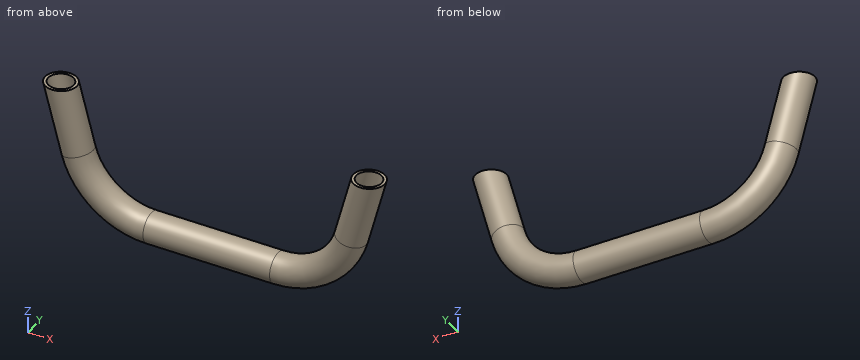
```python
from build123d import *

# Parameters (mm, degrees)
F2_R          = 10
F2_R_2        = 8
F4_W          = 386.4285405924
F4_H          = 84.6193959536
F5_DEPTH      = 10.0010001
F5_DEPTH_BACK = 10.0010001


with BuildPart() as f3:
    # F3: sweep along a path in F0
    with BuildLine(Plane.XZ) as f3_path:
        Line((26.7949192431, 100), (9.9299419155, 37.0590477449))
        ThreePointArc((9.9299419155, 37.0590477449), (-7.9282779485, 10.3323329854), (-38.3663493989, 0))
        Line((-38.3663493989, 0), (-121.7617798121, 0))
        ThreePointArc((-121.7617798121, 0), (-152.1998512625, 10.3323329854), (-170.0580711265, 37.0590477449))
        Line((-170.0580711265, 37.0590477449), (-186.9230484541, 100))
    # F2 (on line) → F3 (sweep)
    with BuildSketch(Plane(origin=(26.7949192431, 0, 100), x_dir=(0.9659258263, 0, -0.2588190451), z_dir=(0.2588190451, 0, 0.9659258263))):
        Circle(F2_R)
        Circle(F2_R_2, mode=Mode.SUBTRACT)
    sweep(path=f3_path.line)

    # F4 (on Front) → F5 (cut, two sides)
    with BuildSketch(Plane.XZ) as f5_sk:
        with Locations((-98.1307812035, 122.3096979768)):
            Rectangle(F4_W, F4_H)
    extrude(amount=-F5_DEPTH, mode=Mode.SUBTRACT)
    extrude(f5_sk.sketch, amount=F5_DEPTH_BACK, mode=Mode.SUBTRACT)


solid = f3.part
```
Part model, mm, in its own coordinate system. Give positions to 0.01 mm unless a question says otherwise; leave off trailing zeros. Order: outer loops, then holes, each group sorted by start corner. A loop starts at its lowest first (then second) coordinate and runs counter-clockwise, first axis right, second up. Notation, with made-up numbers: M 77.5,6.5 L 124.5,6.5 A21 cw 124.5,37.5 Z; hole C 22.5,52.25 d7. An arc over 180 degrees is marked long. Use a Markdown table: item, result. Add a question column.
(1) Saw through at C-C, the plane z = 16.5. Give the number of separate pieces and of enclosed holes in the cut face, and give its area (3 significant figures).
(2) Saw through at A-A, the plane y = 2. Give the cut face in (x, z), and give its area (3 significant figures).
(3) Drop flat-ended pins along their axis: P1, Ø6, axis at y = 5, z = 44, coming from the +X side; P2, Ø9.5, axis at y = 0, z = 0, coming from the -X side; P3, Ø3, axis at y = -6, z = 34, coming from the +X side. Give the stop position or say it passes through.
(4) Probe line 1 along Z through (x, y) = (-67.5, 0); line 2 along Y through (x, z) = (-9.5, 8.5); line 3 along X through (y, z) = (1.25, 32). List the from-to ranges inside material, lowest first. Write a range as [from, to].
(5) Saw through at B-B, the plane x = -70. Give the cut face in (y, z).
Answer key:
| question | item | result |
|---|---|---|
| 1 | separate pieces | 2 |
| 1 | enclosed holes | 2 |
| 1 | area | 318 mm^2 |
| 2 | outline | M -191.71,80 L -179.52,34.52 A59.8 ccw -121.76,-9.8 L -38.37,-9.8 A59.8 ccw 19.39,34.52 L 31.58,80 L 29.46,80 L 17.41,35.05 A57.75 cw -38.37,-7.75 L -121.76,-7.75 A57.75 cw -177.54,35.05 L -189.58,80 Z; M -173.54,80 L -162.58,39.06 A42.25 ccw -121.76,7.75 L -38.37,7.75 A42.25 ccw 2.45,39.06 L 13.42,80 L 11.29,80 L 0.47,39.59 A40.2 cw -38.37,9.8 L -121.76,9.8 A40.2 cw -160.59,39.59 L -171.42,80 Z |
| 2 | area | 1,240 mm^2 |
| 3 | P1 | x = 22.28 |
| 3 | P2 | x = -161.16 |
| 3 | P3 | x = 18.45 |
| 4 | line 1 | [-10, -8], [8, 10] |
| 4 | line 2 | [-9.98, -7.98], [7.98, 9.98] |
| 4 | line 3 | [-178.92, -176.79], [-159.82, -157.57], [-2.56, -0.31], [16.67, 18.79] |
| 5 | outline | C 0,0 d20; hole C 0,0 d16 |
